Could you check a few things on this model? Use its own coordinates, in mm. Round coordinates to 2 decimals unless told otherwise and drop trailing zeros. Loops run counter-clockwise (first coordinate to the right, second up) from the corner with the lowest first, then second, coordinate; pieces in that order, holes last. Notation, with made-up numbers: (2.25, -19.5) -> (54.25, -19.5) arc R8 cw to (54.25, -14.5) -> close; hole circle Ø5 at (56.5, -35.5). An arc over 180 degrees is marked (long way). One line per item, written item: value.
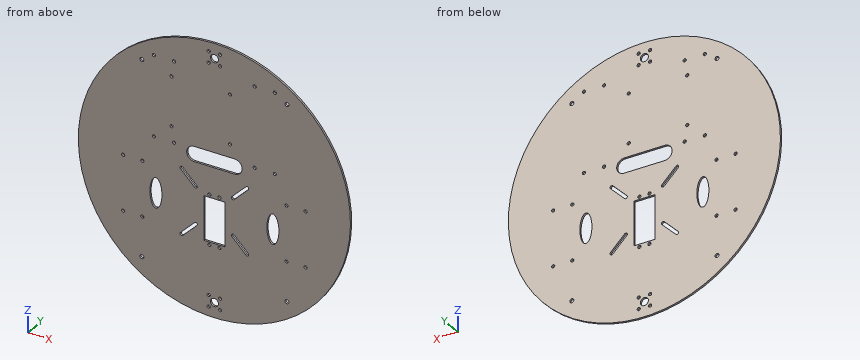
from build123d import *

# Parameters (mm, degrees)
SKETCH_1_R          = 135
EXTRUDE_1_DEPTH     = 2
SKETCH_562_R        = 1.6
SKETCH_562_W        = 21
SKETCH_562_H        = 44
CUT_EXTRUDE_1_DEPTH = 10
SKETCH_1031_R       = 1.6
CUT_EXTRUDE_2_DEPTH = 10
SKETCH_4_R          = 2
SKETCH_4_R_2        = 4
SKETCH_4_R_3        = 1.6
CUT_EXTRUDE_3_DEPTH = 10
CUT_EXTRUDE_4_DEPTH = 10
SKETCH_6_R          = 1.6
SKETCH_6_RX         = 15
SKETCH_6_RY         = 6
CUT_EXTRUDE_7_DEPTH = 10


with BuildPart() as part:
    # 草图1 → 凸台-拉伸1 (new body)
    with BuildSketch(Plane(origin=(0, 0, 0), x_dir=(1, 0, 0), z_dir=(0, 1, 0))):
        with Locations(Location((0, 0, 0), (0, 0, 270))):
            Circle(SKETCH_1_R)
    extrude(amount=EXTRUDE_1_DEPTH)

    # Sketch 562 → 切除-拉伸1 (cut)
    with BuildSketch(Plane(origin=(0, 2, 0), x_dir=(1, 0, 0), z_dir=(0, 1, 0))):
        with Locations(Location((-5, 64.75, 0), (0, 0, 270))):
            Circle(SKETCH_562_R)
        with Locations(Location((5, 64.75, 0), (0, 0, 270))):
            Circle(SKETCH_562_R)
        with Locations(Location((-5, 15.25, 0), (0, 0, 270))):
            Circle(SKETCH_562_R)
        with Locations(Location((5, 15.25, 0), (0, 0, 270))):
            Circle(SKETCH_562_R)
        with Locations(Location((18.5, 48.5, 0), (0, 0, 270))):
            Circle(SKETCH_562_R)
        with Locations(Location((18.5, 11.5, 0), (0, 0, 270))):
            Circle(SKETCH_562_R)
        with Locations(Location((-18.5, 11.5, 0), (0, 0, 270))):
            Circle(SKETCH_562_R)
        with Locations(Location((-18.5, 48.5, 0), (0, 0, 270))):
            Circle(SKETCH_562_R)
        with Locations((0, 40)):
            Rectangle(SKETCH_562_W, SKETCH_562_H)
    extrude(amount=-CUT_EXTRUDE_1_DEPTH, mode=Mode.SUBTRACT)

    # Sketch 1031 → 切除-拉伸2 (cut)
    with BuildSketch(Plane(origin=(0, 2, 0), x_dir=(1, 0, 0), z_dir=(0, 1, 0))):
        with Locations(Location((-60, -25, 0), (0, 0, 270))):
            Circle(SKETCH_1031_R)
        with Locations(Location((-40, -25, 0), (0, 0, 270))):
            Circle(SKETCH_1031_R)
        with Locations(Location((40, -25, 0), (0, 0, 270))):
            Circle(SKETCH_1031_R)
        with Locations(Location((60, -25, 0), (0, 0, 270))):
            Circle(SKETCH_1031_R)
        with Locations(Location((60, -105, 0), (0, 0, 270))):
            Circle(SKETCH_1031_R)
        with Locations(Location((40, -105, 0), (0, 0, 270))):
            Circle(SKETCH_1031_R)
        with Locations(Location((-40, -105, 0), (0, 0, 270))):
            Circle(SKETCH_1031_R)
        with Locations(Location((-60, -105, 0), (0, 0, 270))):
            Circle(SKETCH_1031_R)
        with Locations(Location((-42.5, -89.5, 0), (0, 0, 270))):
            Circle(SKETCH_1031_R)
        with Locations(Location((-42.5, -40.5, 0), (0, 0, 270))):
            Circle(SKETCH_1031_R)
        with Locations(Location((15.5, -40.5, 0), (0, 0, 270))):
            Circle(SKETCH_1031_R)
        with Locations(Location((15.5, -89.5, 0), (0, 0, 270))):
            Circle(SKETCH_1031_R)
    extrude(amount=-CUT_EXTRUDE_2_DEPTH, mode=Mode.SUBTRACT)

    # 草图4 → 切除-拉伸3 (cut)
    with BuildSketch(Plane(origin=(0, 2, 0), x_dir=(1, 0, 0), z_dir=(0, 1, 0))):
        with Locations(Location((-72, 97, 0), (0, 0, 270))):
            Circle(SKETCH_4_R)
        with Locations(Location((72, 97, 0), (0, 0, 270))):
            Circle(SKETCH_4_R)
        with Locations(Location((72, -97, 0), (0, 0, 270))):
            Circle(SKETCH_4_R)
        with Locations(Location((-72, -97, 0), (0, 0, 270))):
            Circle(SKETCH_4_R)
        with Locations(Location((0, -120, 0), (0, 0, 270))):
            Circle(SKETCH_4_R_2)
        with Locations(Location((-5.656854249, -125.656854249, 0), (0, 0, 270))):
            Circle(SKETCH_4_R_3)
        with Locations(Location((-5.656854249, -114.343145751, 0), (0, 0, 270))):
            Circle(SKETCH_4_R_3)
        with Locations(Location((5.656854249, -114.343145751, 0), (0, 0, 270))):
            Circle(SKETCH_4_R_3)
        with Locations(Location((5.656854249, -125.656854249, 0), (0, 0, 270))):
            Circle(SKETCH_4_R_3)
        with Locations(Location((5.656854249, 125.656854249, 0), (0, 0, 270))):
            Circle(SKETCH_4_R_3)
        with Locations(Location((5.656854249, 114.343145751, 0), (0, 0, 270))):
            Circle(SKETCH_4_R_3)
        with Locations(Location((-5.656854249, 114.343145751, 0), (0, 0, 270))):
            Circle(SKETCH_4_R_3)
        with Locations(Location((-5.656854249, 125.656854249, 0), (0, 0, 270))):
            Circle(SKETCH_4_R_3)
        with Locations(Location((0, 120, 0), (0, 0, 270))):
            Circle(SKETCH_4_R_2)
        with BuildLine():
            Line((-20, -12.5), (20, -12.5))
            ThreePointArc((20, -12.5), (27.5, -20), (20, -27.5))
            Line((20, -27.5), (-20, -27.5))
            ThreePointArc((-20, -27.5), (-27.5, -20), (-20, -12.5))
        make_face()
    extrude(amount=-CUT_EXTRUDE_3_DEPTH, mode=Mode.SUBTRACT)

    # 草图5 → 切除-拉伸4 (cut)
    with BuildSketch(Plane(origin=(0, 2, 0), x_dir=(1, 0, 0), z_dir=(0, 1, 0))):
        with BuildLine():
            Line((-31.36862915, 63.63137085), (-17.36862915, 49.63137085))
            ThreePointArc((-17.36862915, 49.63137085), (-17.36862915, 47.36862915), (-19.63137085, 47.36862915))
            Line((-19.63137085, 47.36862915), (-33.63137085, 61.36862915))
            ThreePointArc((-33.63137085, 61.36862915), (-33.63137085, 63.63137085), (-31.36862915, 63.63137085))
        make_face()
        with BuildLine():
            Line((33.63137085, 61.36862915), (19.63137085, 47.36862915))
            ThreePointArc((19.63137085, 47.36862915), (17.36862915, 47.36862915), (17.36862915, 49.63137085))
            Line((17.36862915, 49.63137085), (31.36862915, 63.63137085))
            ThreePointArc((31.36862915, 63.63137085), (33.63137085, 63.63137085), (33.63137085, 61.36862915))
        make_face()
        with BuildLine():
            Line((31.36862915, -3.63137085), (17.36862915, 10.36862915))
            ThreePointArc((17.36862915, 10.36862915), (17.36862915, 12.63137085), (19.63137085, 12.63137085))
            Line((19.63137085, 12.63137085), (33.63137085, -1.36862915))
            ThreePointArc((33.63137085, -1.36862915), (33.63137085, -3.63137085), (31.36862915, -3.63137085))
        make_face()
        with BuildLine():
            Line((-33.63137085, -1.36862915), (-19.63137085, 12.63137085))
            ThreePointArc((-19.63137085, 12.63137085), (-17.36862915, 12.63137085), (-17.36862915, 10.36862915))
            Line((-17.36862915, 10.36862915), (-31.36862915, -3.63137085))
            ThreePointArc((-31.36862915, -3.63137085), (-33.63137085, -3.63137085), (-33.63137085, -1.36862915))
        make_face()
    extrude(amount=-CUT_EXTRUDE_4_DEPTH, mode=Mode.SUBTRACT)

    # 草图6 → 切除-拉伸7 (cut)
    with BuildSketch(Plane(origin=(0, 2, 0), x_dir=(1, 0, 0), z_dir=(0, 1, 0))):
        with Locations(Location((71.537199543, 2.5, 0), (0, 0, 270))):
            Circle(SKETCH_6_R)
        with Locations(Location((90.537199543, 2.5, 0), (0, 0, 270))):
            Circle(SKETCH_6_R)
        with Locations(Location((90.537199543, 57.5, 0), (0, 0, 270))):
            Circle(SKETCH_6_R)
        with Locations(Location((71.537199543, 57.5, 0), (0, 0, 270))):
            Circle(SKETCH_6_R)
        with Locations(Location((-71.537199543, 57.5, 0), (0, 0, 270))):
            Circle(SKETCH_6_R)
        with Locations(Location((-90.537199543, 2.5, 0), (0, 0, 270))):
            Circle(SKETCH_6_R)
        with Locations(Location((-71.537199543, 2.5, 0), (0, 0, 270))):
            Circle(SKETCH_6_R)
        with Locations(Location((-90.537199543, 57.5, 0), (0, 0, 270))):
            Circle(SKETCH_6_R)
        with Locations(Location((-58.031053316, 30), (0, 0, -90))):
            Ellipse(SKETCH_6_RX, SKETCH_6_RY)
        with Locations(Location((58.031053316, 30), (0, 0, 90))):
            Ellipse(SKETCH_6_RX, SKETCH_6_RY)
    extrude(amount=-CUT_EXTRUDE_7_DEPTH, mode=Mode.SUBTRACT)


solid = part.part
(1) If we section it at D-D, the plane x = -79: Please give me the cut outline in (y, z), then the cut area to 3 significant figures.
Recorded:
outline: (0, -109.47) -> (2, -109.47) -> (2, 109.47) -> (0, 109.47) -> close
area: 438 mm²
(2) If we section it at A-A, the plane z = -120: Please give me the cut outline in (x, y).
Recorded:
outline: (-61.85, 0) -> (-4, 0) -> (-4, 2) -> (-61.85, 2) -> close; (4, 0) -> (61.85, 0) -> (61.85, 2) -> (4, 2) -> close
(3) If I drill on L1, parallel to X at y = 1.95, z = -65; L2, parallel to Z at x = 17.5, y = 1.35; L3, parallel to X at y = 0.65, z = -42, over which ranges is the centre line in solid material (lowest first)?
Recorded:
L1: -118.32 to -6.58, -3.42 to 3.42, 6.58 to 118.32
L2: -133.86 to -49.76, -47.25 to -12.75, -10.24 to 12.5, 27.5 to 133.86
L3: -128.3 to -61.63, -54.43 to -10.5, 10.5 to 54.43, 61.63 to 128.3
(4) If we section it at C-C, the plane x = 98: Please give me the cut outline in (y, z).
Recorded:
outline: (0, -92.85) -> (2, -92.85) -> (2, 92.85) -> (0, 92.85) -> close
(5) If we section it at B-B, the plane y = 0.7: Give the number of separate pieces and of enclosed holes in the cut face, then the cut area to 3 significant figures.
Recorded:
separate pieces: 1
enclosed holes: 46
area: 54,300 mm²
(6) I'm going to push a flat-ended pin straight in: pin 1 Ø3.5 at (x, z) = (-72, -97) entering from -Y. Where does the tip first touch, or does it pass through?
Recorded:
pin 1: through
